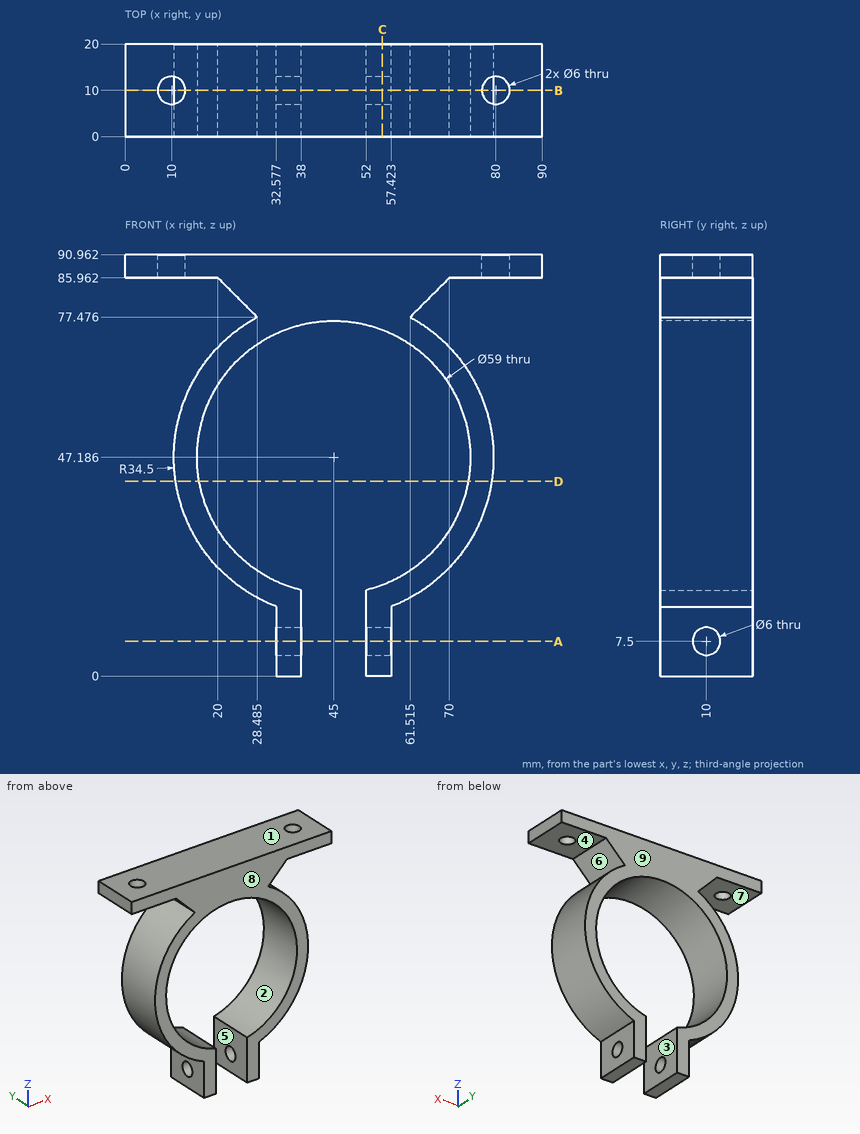
The drawing under review shows one solid part. Ordinate dimensions are in mm from its lowest x, y, z. A direction names the side the tool comes from. Round coordinates to 2 decimals unless told otherwise and drop trailing zeros. Write each loop counter-clockwise with the first axis right and the second up, starting at its lowest first coordinate (ties: lowest second). Pieces come first, ordered by that corner, then holes.
(1) We need section A-A on z = 7.5. Give the boundary of the cut face in (x, y), and give its area (3 significant figures).
(2) Wall thickness on L1, parallel to X at y = 10, z = 87.7; L2, parallel to Y at x = 34.35, z = 7.5; L3, parallel to Z at x = 21.5, y = 7.25 (1 decimal): over which ranges is each line inside the solid? List them lowest first.
(3) We need section B-B on y = 10. Give the number of separate pieces and of enclosed holes in the cut face, and give its area (3 significant figures).
(4) Insertion check: pin 1 (1.5 mm diameter, centred on x = 25, y = 6, fed in from -Z) (1 decimal); pin 2 (12 mm diameter, centred on y = 14.5, z = 4, fed in from +X); pin 3 (5 mm diameter, centred on x = 28.5, y = 11, fed in from -Z) (1 decimal); pin 4 (12 mm diameter, centred on x = 32, y = 6.5, fed in from -Z). Each pin has a flat end and moves straight along its axis. Give the tip position at first contact, or say it passes through.
(5) Mouldability with a two-part tool opening along Z and no side actions: class the marked faces 1, 2, 3 and 4 as +Z half, -Z half, draft (parallel to the pull), parting line (faces both ways), or undercut.
(6) We need section C-C on x = 55.5. Give the boundary of the cut face in (y, z), and give its area (3 significant figures).
(7) Machinability: for the marked faces 5, 6, 7, 8 and 9, which of the approach directions +Z, -Z, +X, -X, +Y, -Y give a long, thin tool a straight path to every point of the face, cutting with its end or side? Answer none if there is none.
(8) We need section D-D on z = 42. Give the boundary of the cut face in (x, y).
Findings below:
1. outline: (32.58, 0) - (38, 0) - (38, 7) - (32.58, 7) - close; (32.58, 13) - (38, 13) - (38, 20) - (32.58, 20) - close; (52, 0) - (57.42, 0) - (57.42, 7) - (52, 7) - close; (52, 13) - (57.42, 13) - (57.42, 20) - (52, 20) - close
1. area: 152 mm2
2. L1: x = 0 to 7, 13 to 77, 83 to 90
2. L2: y = 0 to 7, 13 to 20
2. L3: z = 21.9 to 29.4, 65 to 72.4, 84.5 to 91
3. separate pieces: 5
3. enclosed holes: 0
3. area: 1,670 mm2
4. pin 1: stops at z = 18.6
4. pin 2: stops at x = 57.42
4. pin 3: stops at z = 15.7
4. pin 4: stops at z = 0
5. face 1: +Z half
5. face 2: undercut
5. face 3: draft
5. face 4: undercut
6. outline: (0, 0) - (20, 0) - (20, 19.62) - (0, 19.62) - close; (0, 74.75) - (20, 74.75) - (20, 90.96) - (0, 90.96) - close; hole circle Ø6 at (10, 7.5)
6. area: 688 mm2
7. face 5: -Z, +Y, -Y
7. face 6: +X, +Y, -Y
7. face 7: -X, +Y, -Y
7. face 8: +Z, -Z, +X, -X, -Y
7. face 9: +Z, -Z, +X, -X, +Y
8. outline: (10.89, 0) - (15.96, 0) - (15.96, 20) - (10.89, 20) - close; (74.04, 0) - (79.11, 0) - (79.11, 20) - (74.04, 20) - close
